Geometry: final body of the model. Coordinates: model frame, mm. Round coordinates to 2 decimals unless told otherwise and drop trailing zeros. Loops run counter-clockwise (first coordinate to the right, second up) from the corner with the lowest first, then second, coordinate; pieces in that order, holes last. Notation, with made-up numbers: M 15,65 L 35,65 A21 ccw 35,89 Z; hole C -8.5,7.25 d4. An arc over 180 degrees is marked long. Answer as a JSON object with one key per item and string values.
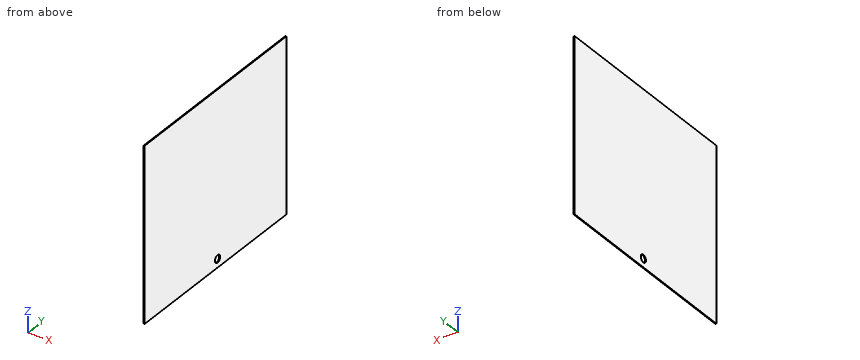
```python
from build123d import *

# Parameters (mm, degrees)
CROQUIS1_W              = 580
CROQUIS1_H              = 680
SALIENTE_EXTRUIR1_DEPTH = 3
CORTAR_EXTRUIR1_REACH   = 448.888
CROQUIS2_R              = 12.5


with BuildPart() as part:
    # Croquis1 → Saliente-Extruir1 (new body)
    with BuildSketch(Plane(origin=(0, 0, 0), x_dir=(0, 0, -1), z_dir=(1, 0, 0))):
        Rectangle(CROQUIS1_W, CROQUIS1_H)
    extrude(amount=SALIENTE_EXTRUIR1_DEPTH)

    # Croquis2 → Cortar-Extruir1 (cut, up to next)
    with BuildSketch(Plane.ZY, mode=Mode.PRIVATE) as cortar_extruir1_sk1:
        with Locations((-261.5, 10)):
            Circle(CROQUIS2_R)
    cortar_extruir1_tool1 = extrude(cortar_extruir1_sk1.sketch, amount=-CORTAR_EXTRUIR1_REACH, mode=Mode.PRIVATE) & part.part
    add(cortar_extruir1_tool1.solids().sort_by_distance((0, 10, -261.5))[0], mode=Mode.SUBTRACT)


solid = part.part
```
1) Line query: probe 1 along Y at (x, z) = (1, -261.5); probe 2 along Z at (x, y) = (0.9, 21.5). Output: solid intervals per line, ascending.
Geometry results:
{"probe 1": "-340 to -2.5, 22.5 to 340", "probe 2": "-290 to -266.4, -256.6 to 290"}
2) Cut plane A-A on y = 10. Return the cut outline in (x, z), and give its area (4 significant figures).
Geometry results:
{"outline": "M 0,-290 L 3,-290 L 3,-274 L 0,-274 Z; M 0,-249 L 3,-249 L 3,290 L 0,290 Z", "area": "1,665 mm2"}
3) Cut plane B-B on z = -261.5. Return the cut outline in (x, y).
Geometry results:
{"outline": "M 0,-340 L 3,-340 L 3,-2.5 L 0,-2.5 Z; M 0,22.5 L 3,22.5 L 3,340 L 0,340 Z"}
4) First-contact query: pin 1 (1 mm diameter, centred on y = -270, z = 65.5, fed in from -X). Flat tip, straight axial feed; report the tip coordinate or a pass-through.
Geometry results:
{"pin 1": "x = 0"}
